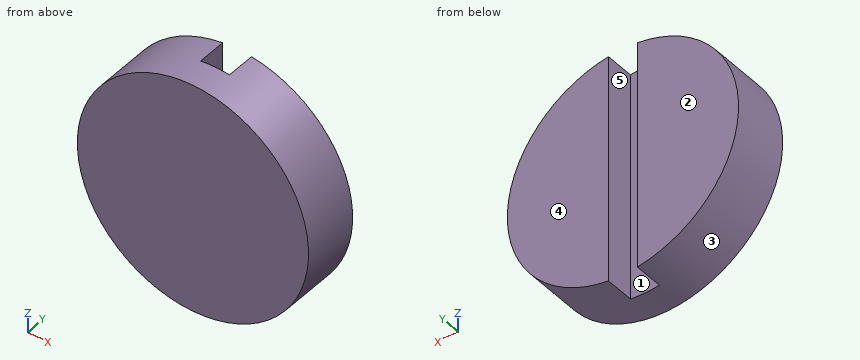
```python
from build123d import *

# Parameters (mm, degrees)
CROQUIS1_R              = 4
SALIENTE_EXTRUIR1_DEPTH = 2
CORTAR_EXTRUIR1_START   = -1
CORTAR_EXTRUIR1_DEPTH   = 1


with BuildPart() as part:
    # Croquis1 → Saliente-Extruir1 (new body)
    with BuildSketch(Plane(origin=(0, 0, 0), x_dir=(1, 0, 0), z_dir=(0, 1, 0))):
        with Locations(Location((0, 0, 0), (0, 0, 270))):
            Circle(CROQUIS1_R)
    extrude(amount=SALIENTE_EXTRUIR1_DEPTH)

    # Croquis2 → Cortar-Extruir1 (cut)
    with BuildSketch(Plane(origin=(0, 2, 0), x_dir=(1, 0, 0), z_dir=(0, 1, 0)).offset(CORTAR_EXTRUIR1_START)):
        with BuildLine():
            Line((-0.5, 3.968626967), (-0.5, -3.968626967))
            ThreePointArc((-0.5, -3.968626967), (0, -4), (0.5, -3.968626967))
            Line((0.5, -3.968626967), (0.5, 3.968626967))
            ThreePointArc((0.5, 3.968626967), (0, 4), (-0.5, 3.968626967))
        make_face()
    extrude(amount=CORTAR_EXTRUIR1_DEPTH, mode=Mode.SUBTRACT)


solid = part.part
```
Check sheet for the modelled part. Datum: model origin and axes. Units: mm. Face numbers are marked on the shaded views. A direction names the side the tool comes from. Coordinates: 2 decimals unless noted, no trailing zeros. Order: outer loops, then holes, each group sorted by start corner. A loop starts at its lowest first (then second) coordinate and runs counter-clockwise, first axis right, second up. Notation, with made-up numbers: M -32,-11.75 L 11,-11.75 A14 cw 11,14.25 Z; hole C -32,26 d3. An arc over 180 degrees is marked long. Write each question's results on one line, items separated by ' | '. Start each with the question number.
1. Cross-section at D-D on z = -3.5. Record the cut outline in (x, y).
2. Cross-section at C-C on x = 0. Record the cut outline in (y, z), and give its area (3 significant figures).
3. Go/stop test with flat-tipped pins: P1, Ø1.1, axis at y = 1.5, z = 1, coming from the -X side; P2, Ø1, axis at x = 1, y = 1.5, coming from the +Z side; P3, Ø0.5, axis at y = 1.5, z = -1, coming from the +X side. Record where each tip stops, or that it passes through.
4. Material ranges on probe 1 along X at (y, z) = (1.65, 3); probe 2 along X at (y, z) = (1.15, 0.5); probe 3 along Y at (x, z) = (0, -3.25), recorded low to high.
5. Mould release check, pull along X, two halves, no side actions. Record for the marked faces 1, 2 and 3: +X half, -X half, draft (parallel to the pull), parting line (faces both ways), or undercut.
6. Cross-section at A-A on z = 0. Record the cut outline in (x, y), and give its area (3 significant figures).
7. Cross-section at B-B on y = 1.4. Record the cut outline in (x, z), and give its area (3 significant figures).
8. Access from +Z, -Z, +X, -X, +Y, -Y to the whole of each face (thin tool, end or side, straight path). Record for the marked faces 4 and 5.
Checks:
1) outline: M -1.94,0 L 1.94,0 L 1.94,2 L 0.5,2 L 0.5,1 L -0.5,1 L -0.5,2 L -1.94,2 Z
2) outline: M 0,-4 L 1,-4 L 1,4 L 0,4 Z | area: 8.00 mm²
3) P1: stops at x = -3.97 | P2: stops at z = 3.97 | P3: stops at x = 3.93
4) probe 1: x = -2.65 to -0.5, 0.5 to 2.65 | probe 2: x = -3.97 to -0.5, 0.5 to 3.97 | probe 3: y = 0 to 1
5) face 1: undercut | face 2: draft | face 3: parting line
6) outline: M -4,0 L 4,0 L 4,2 L 0.5,2 L 0.5,1 L -0.5,1 L -0.5,2 L -4,2 Z | area: 15.0 mm²
7) outline: M -0.5,-3.97 L -0.5,3.97 A4 ccw Z; M 0.5,-3.97 A4 ccw 0.5,3.97 Z | area: 42.3 mm²
8) face 4: +Z, -Z, +X, -X, +Y | face 5: +Z, -Z, +Y
